CAD build for the part. Positions are in the model's coordinates, mm. A direction names the side the tool comes from. Give positions to 0.01 mm unless a question says otherwise; leave off trailing zeros. Loops run counter-clockwise (first coordinate to the right, second up) from the corner with the lowest first, then second, coordinate; pieces in that order, holes last. Notation, with made-up numbers: (76, 25) -> (102, 25) arc R30 cw to (102, 59) -> close; hole circle Ø5 at (71.5, -20.75). An arc over 180 degrees is marked (long way). Use one line per item in the form item = value.
```python
from build123d import *

# Parameters (mm, degrees)
SKETCH1_R                       = 27
SKETCH1_R_2                     = 1.05
BOSS_EXTRUDE1_DEPTH             = 3
SKETCH2_R                       = 27
SKETCH2_R_2                     = 12
BOSS_EXTRUDE2_DEPTH             = 1.65
SKETCH3_R                       = 27
SKETCH3_R_2                     = 15.15
BOSS_EXTRUDE3_DEPTH             = 5
BOSS_EXTRUDE4_START             = 3
SKETCH4_R                       = 27
SKETCH4_R_2                     = 1.875
BOSS_EXTRUDE4_DEPTH             = 3
SKETCH6_R                       = 1.25
CUT_EXTRUDE2_DEPTH              = 41.224650402
CIRPATTERN2_COUNT               = 4
BOSS_EXTRUDE5_REACH             = 41.384
BOSS_EXTRUDE5_DIRECTION_2_REACH = 41.384


with BuildPart() as part:
    # Sketch1 → Boss-Extrude1 (new body)
    with BuildSketch(Plane(origin=(0, 0, 0), x_dir=(1, 0, 0), z_dir=(0, 1, 0))):
        with Locations(Location((0, 0, 0), (0, 0, 270))):
            Circle(SKETCH1_R)
        with Locations(Location((0, 7, 0), (0, 0, 270))):
            Circle(SKETCH1_R_2, mode=Mode.SUBTRACT)
        with Locations(Location((0, -7, 0), (0, 0, 270))):
            Circle(SKETCH1_R_2, mode=Mode.SUBTRACT)
    extrude(amount=BOSS_EXTRUDE1_DEPTH)

    # Sketch2 → Boss-Extrude2 (add)
    with BuildSketch(Plane(origin=(0, 3, 0), x_dir=(1, 0, 0), z_dir=(0, 1, 0))):
        with Locations(Location((0, 0, 0), (0, 0, 270))):
            Circle(SKETCH2_R)
        with Locations(Location((0, 0, 0), (0, 0, 270))):
            Circle(SKETCH2_R_2, mode=Mode.SUBTRACT)
    extrude(amount=BOSS_EXTRUDE2_DEPTH)

    # Sketch3 → Boss-Extrude3 (add)
    with BuildSketch(Plane(origin=(0, 4.65, 0), x_dir=(1, 0, 0), z_dir=(0, 1, 0))):
        with Locations(Location((0, 0, 0), (0, 0, 270))):
            Circle(SKETCH3_R)
        with Locations(Location((0, 0, 0), (0, 0, 270))):
            Circle(SKETCH3_R_2, mode=Mode.SUBTRACT)
    extrude(amount=BOSS_EXTRUDE3_DEPTH)

    # Sketch4 → Boss-Extrude4 (add)
    with BuildSketch(Plane.XZ.offset(BOSS_EXTRUDE4_START)):
        with Locations(Location((0, 0, 0), (0, 0, 270))):
            Circle(SKETCH4_R)
        with Locations(Location((0, -7, 0), (0, 0, 270))):
            Circle(SKETCH4_R_2, mode=Mode.SUBTRACT)
        with Locations(Location((0, 7, 0), (0, 0, 270))):
            Circle(SKETCH4_R_2, mode=Mode.SUBTRACT)
    extrude(amount=-BOSS_EXTRUDE4_DEPTH)

    # Sketch6 → Cut-Extrude2 (cut, through all)
    with BuildSketch(Plane(origin=(0, 9.65, 0), x_dir=(1, 0, 0), z_dir=(0, 1, 0))):
        with Locations(Location((0, 23.5, 0), (0, 0, 270))):
            Circle(SKETCH6_R)
    cut_extrude2 = extrude(amount=-CUT_EXTRUDE2_DEPTH, mode=Mode.SUBTRACT)

    # CirPattern2: Cut-Extrude2 ×4 about axis
    cirpattern2_axis = Axis((0, 0, 0), (0, 1, 0))
    for i in range(1, CIRPATTERN2_COUNT):
        add(cut_extrude2.rotate(cirpattern2_axis, i * 360 / CIRPATTERN2_COUNT), mode=Mode.SUBTRACT)

    # Boss-Extrude5: up to this face of the body (flat: up to its plane)
    boss_extrude5_end = Plane(part.part.faces().sort_by_distance((0, 9.65, -26.236324676))[0])
    # Sketch7 → Boss-Extrude5 (add, up to the picked face)
    with BuildSketch(Plane(origin=(0, 0, 0), x_dir=(1, 0, 0), z_dir=(0, 1, 0)), mode=Mode.PRIVATE) as boss_extrude5_sk1:
        with BuildLine():
            Line((0, 27), (-27, 27))
            Line((-27, 27), (-27, 0))
            ThreePointArc((-27, 0), (-19.091883092, 19.091883092), (0, 27))
        make_face()
    boss_extrude5_tool1 = split(extrude(boss_extrude5_sk1.sketch, amount=BOSS_EXTRUDE5_REACH, mode=Mode.PRIVATE), bisect_by=boss_extrude5_end, keep=Keep.BOTH, mode=Mode.PRIVATE)
    # Sketch7 → Boss-Extrude5 (add, up to the picked face)
    with BuildSketch(Plane(origin=(0, 0, 0), x_dir=(1, 0, 0), z_dir=(0, 1, 0)), mode=Mode.PRIVATE) as boss_extrude5_sk2:
        with BuildLine():
            Line((27, 27), (0, 27))
            ThreePointArc((0, 27), (19.091883092, 19.091883092), (27, 0))
            Line((27, 0), (27, 27))
        make_face()
    boss_extrude5_tool2 = split(extrude(boss_extrude5_sk2.sketch, amount=BOSS_EXTRUDE5_REACH, mode=Mode.PRIVATE), bisect_by=boss_extrude5_end, keep=Keep.BOTH, mode=Mode.PRIVATE)
    # Sketch7 → Boss-Extrude5 (add, up to the picked face)
    with BuildSketch(Plane(origin=(0, 0, 0), x_dir=(1, 0, 0), z_dir=(0, 1, 0)), mode=Mode.PRIVATE) as boss_extrude5_sk3:
        with BuildLine():
            Line((27, -27), (27, 0))
            ThreePointArc((27, 0), (19.091883057, -19.091883127), (-9.8e-08, -27))
            Line((-9.8e-08, -27), (27, -27))
        make_face()
    boss_extrude5_tool3 = split(extrude(boss_extrude5_sk3.sketch, amount=BOSS_EXTRUDE5_REACH, mode=Mode.PRIVATE), bisect_by=boss_extrude5_end, keep=Keep.BOTH, mode=Mode.PRIVATE)
    # Sketch7 → Boss-Extrude5 (add, up to the picked face)
    with BuildSketch(Plane(origin=(0, 0, 0), x_dir=(1, 0, 0), z_dir=(0, 1, 0)), mode=Mode.PRIVATE) as boss_extrude5_sk4:
        with BuildLine():
            ThreePointArc((-9.8e-08, -27), (-19.091883127, -19.091883057), (-27, 0))
            Line((-27, 0), (-27, -27))
            Line((-27, -27), (-9.8e-08, -27))
        make_face()
    boss_extrude5_tool4 = split(extrude(boss_extrude5_sk4.sketch, amount=BOSS_EXTRUDE5_REACH, mode=Mode.PRIVATE), bisect_by=boss_extrude5_end, keep=Keep.BOTH, mode=Mode.PRIVATE)
    add(boss_extrude5_tool1.solids().sort_by(Axis((-20.969066, 0, -20.969066), (0, 1, 0)))[0])
    add(boss_extrude5_tool2.solids().sort_by(Axis((20.969066, 0, -20.969066), (0, 1, 0)))[0])
    add(boss_extrude5_tool3.solids().sort_by(Axis((20.969066, 0, 20.969066), (0, 1, 0)))[0])
    add(boss_extrude5_tool4.solids().sort_by(Axis((-20.969066, 0, 20.969066), (0, 1, 0)))[0])

    # Boss-Extrude5 direction 2: up to this face of the body (flat: up to its plane)
    boss_extrude5_direction_2_end = Plane(part.part.faces().sort_by_distance((0, -3, 0))[0])
    # Sketch7 → Boss-Extrude5 direction 2 (add, up to the picked face)
    with BuildSketch(Plane(origin=(0, 0, 0), x_dir=(1, 0, 0), z_dir=(0, 1, 0)), mode=Mode.PRIVATE) as boss_extrude5_direction_2_sk1:
        with BuildLine():
            Line((0, 27), (-27, 27))
            Line((-27, 27), (-27, 0))
            ThreePointArc((-27, 0), (-19.091883092, 19.091883092), (0, 27))
        make_face()
    boss_extrude5_direction_2_tool1 = split(extrude(boss_extrude5_direction_2_sk1.sketch, amount=-BOSS_EXTRUDE5_DIRECTION_2_REACH, mode=Mode.PRIVATE), bisect_by=boss_extrude5_direction_2_end, keep=Keep.BOTH, mode=Mode.PRIVATE)
    # Sketch7 → Boss-Extrude5 direction 2 (add, up to the picked face)
    with BuildSketch(Plane(origin=(0, 0, 0), x_dir=(1, 0, 0), z_dir=(0, 1, 0)), mode=Mode.PRIVATE) as boss_extrude5_direction_2_sk2:
        with BuildLine():
            Line((27, 27), (0, 27))
            ThreePointArc((0, 27), (19.091883092, 19.091883092), (27, 0))
            Line((27, 0), (27, 27))
        make_face()
    boss_extrude5_direction_2_tool2 = split(extrude(boss_extrude5_direction_2_sk2.sketch, amount=-BOSS_EXTRUDE5_DIRECTION_2_REACH, mode=Mode.PRIVATE), bisect_by=boss_extrude5_direction_2_end, keep=Keep.BOTH, mode=Mode.PRIVATE)
    # Sketch7 → Boss-Extrude5 direction 2 (add, up to the picked face)
    with BuildSketch(Plane(origin=(0, 0, 0), x_dir=(1, 0, 0), z_dir=(0, 1, 0)), mode=Mode.PRIVATE) as boss_extrude5_direction_2_sk3:
        with BuildLine():
            Line((27, -27), (27, 0))
            ThreePointArc((27, 0), (19.091883057, -19.091883127), (-9.8e-08, -27))
            Line((-9.8e-08, -27), (27, -27))
        make_face()
    boss_extrude5_direction_2_tool3 = split(extrude(boss_extrude5_direction_2_sk3.sketch, amount=-BOSS_EXTRUDE5_DIRECTION_2_REACH, mode=Mode.PRIVATE), bisect_by=boss_extrude5_direction_2_end, keep=Keep.BOTH, mode=Mode.PRIVATE)
    # Sketch7 → Boss-Extrude5 direction 2 (add, up to the picked face)
    with BuildSketch(Plane(origin=(0, 0, 0), x_dir=(1, 0, 0), z_dir=(0, 1, 0)), mode=Mode.PRIVATE) as boss_extrude5_direction_2_sk4:
        with BuildLine():
            ThreePointArc((-9.8e-08, -27), (-19.091883127, -19.091883057), (-27, 0))
            Line((-27, 0), (-27, -27))
            Line((-27, -27), (-9.8e-08, -27))
        make_face()
    boss_extrude5_direction_2_tool4 = split(extrude(boss_extrude5_direction_2_sk4.sketch, amount=-BOSS_EXTRUDE5_DIRECTION_2_REACH, mode=Mode.PRIVATE), bisect_by=boss_extrude5_direction_2_end, keep=Keep.BOTH, mode=Mode.PRIVATE)
    add(boss_extrude5_direction_2_tool1.solids().sort_by(Axis((-20.969066, 0, -20.969066), (0, -1, 0)))[0])
    add(boss_extrude5_direction_2_tool2.solids().sort_by(Axis((20.969066, 0, -20.969066), (0, -1, 0)))[0])
    add(boss_extrude5_direction_2_tool3.solids().sort_by(Axis((20.969066, 0, 20.969066), (0, -1, 0)))[0])
    add(boss_extrude5_direction_2_tool4.solids().sort_by(Axis((-20.969066, 0, 20.969066), (0, -1, 0)))[0])


solid = part.part
```
1. Drill centre lines: line 1 (X direction, y = 6.75, z = -23.5); line 2 (X direction, y = 1.45, z = -7). Where is each one in solid material? Low to high.
Result sheet:
line_1 = -27 to -1.25, 1.25 to 27
line_2 = -27 to -1.05, 1.05 to 27
2. Cut at D-D, the plane x = 5.5. Write the cut outline in (y, z), then the cut area to 3 significant figures.
Result sheet:
outline = (-3, -27) -> (9.65, -27) -> (9.65, -14.12) -> (4.65, -14.12) -> (4.65, -10.67) -> (3, -10.67) -> (3, 10.67) -> (4.65, 10.67) -> (4.65, 14.12) -> (9.65, 14.12) -> (9.65, 27) -> (-3, 27) -> close
area = 507 mm^2
3. Cut at B-B, the plane z = -23.5. Write the cut outline in (x, y).
Result sheet:
outline = (-27, -3) -> (-1.25, -3) -> (-1.25, 9.65) -> (-27, 9.65) -> close; (1.25, -3) -> (27, -3) -> (27, 9.65) -> (1.25, 9.65) -> close
4. Tool access for faces 4 (the cylindrical face through (3.604, 3.813, 11.446)), 5 (the flat face through (0, 3, 27)), 6 (the cylindrical face through (0.082, -1.521, -5.127)): list every direction of +Z, -Z, +X, -X, +Y, -Y with a clear straight run to the whole face (end or side of a thin tool).
Result sheet:
face_4 = +Y
face_5 = +Z, +X, -X, +Y, -Y
face_6 = -Y
5. Cut at A-A, the plane x = -23.5. Write the cut outline in (y, z), then the cut area to 3 significant figures.
Result sheet:
outline = (-3, -27) -> (9.65, -27) -> (9.65, -1.25) -> (-3, -1.25) -> close; (-3, 1.25) -> (9.65, 1.25) -> (9.65, 27) -> (-3, 27) -> close
area = 651 mm^2
6. Drop flat-ended pins along their axis: P1, Ø19, axis at x = 0.5, z = 2, coming from the +Y side; P2, Ø1.9, axis at x = -0.5, z = 7.5, coming from the -Y side. Give the stop position or say it passes through.
Result sheet:
P1 = 3
P2 = 0
7. Mould opens along Z. For faces 1 (the flat face through (27, 3, 0)), 2 (the flat face through (0, 3, -27)), 3 (the cylindrical face through (-0.479, 3.414, -22.345)) say: pulls with the +Z half, pulls with the -Z half, needs draft (parallel to the pull), parting line crosses it, or undercut.
Result sheet:
face_1 = needs draft
face_2 = pulls with the -Z half
face_3 = undercut
8. Cut at C-C, the plane y = 8.25. Write the cut outline in (x, z), then the cut area to 3 significant figures.
Result sheet:
outline = (-27, -27) -> (27, -27) -> (27, 27) -> (-27, 27) -> close; hole circle Ø2.5 at (-23.5, 0); hole circle Ø30.3 at (0, 0); hole circle Ø2.5 at (0, -23.5); hole circle Ø2.5 at (0, 23.5); hole circle Ø2.5 at (23.5, 0)
area = 2,180 mm^2
